```python
from build123d import *

# Parameters (mm, degrees)
SKETCH_1_W            = 100
SKETCH_1_H            = 62
SKETCH_1_W_2          = 110
SKETCH_1_H_2          = 30
EXTRUDE_467_DEPTH     = 2
SKETCH_2_R            = 1.25
CUT_EXTRUDE_872_DEPTH = 2
SKETCH_3_R            = 3.25
SKETCH_3_R_2          = 1.25
EXTRUDE_1188_DEPTH    = 3


with BuildPart() as part:
    # 草图1 → Extrude 467 (new body)
    with BuildSketch(Plane(origin=(0, 0, 0), x_dir=(1, 0, 0), z_dir=(0, 1, 0))):
        Rectangle(SKETCH_1_W, SKETCH_1_H)
        Rectangle(SKETCH_1_W_2, SKETCH_1_H_2)
    extrude(amount=EXTRUDE_467_DEPTH)

    # 草图2 → Cut-Extrude 872 (cut)
    with BuildSketch(Plane(origin=(0, 2, 0), x_dir=(1, 0, 0), z_dir=(0, 1, 0))):
        with Locations((-14, 24.5)):
            Circle(SKETCH_2_R)
        with Locations((44, 24.5)):
            Circle(SKETCH_2_R)
        with Locations((-14, -24.5)):
            Circle(SKETCH_2_R)
        with Locations((44, -24.5)):
            Circle(SKETCH_2_R)
    extrude(amount=-CUT_EXTRUDE_872_DEPTH, mode=Mode.SUBTRACT)

    # 草图3 → Extrude 1188 (add)
    with BuildSketch(Plane(origin=(0, 2, 0), x_dir=(1, 0, 0), z_dir=(0, 1, 0))):
        with Locations((-14, 24.5)):
            Circle(SKETCH_3_R)
        with Locations((-14, 24.5)):
            Circle(SKETCH_3_R_2, mode=Mode.SUBTRACT)
        with Locations((44, 24.5)):
            Circle(SKETCH_3_R)
        with Locations((44, 24.5)):
            Circle(SKETCH_3_R_2, mode=Mode.SUBTRACT)
        with Locations((-14, -24.5)):
            Circle(SKETCH_3_R)
        with Locations((-14, -24.5)):
            Circle(SKETCH_3_R_2, mode=Mode.SUBTRACT)
        with Locations((44, -24.5)):
            Circle(SKETCH_3_R)
        with Locations((44, -24.5)):
            Circle(SKETCH_3_R_2, mode=Mode.SUBTRACT)
    extrude(amount=EXTRUDE_1188_DEPTH)


solid = part.part
```
The listing builds one solid part. Answer for the finished solid, in the listing's coordinates (mm). A direction names the side the tool comes from. Give positions to 0.01 mm unless a question says otherwise; leave off trailing zeros. Order: outer loops, then holes, each group sorted by start corner. A loop starts at its lowest first (then second) coordinate and runs counter-clockwise, first axis right, second up. Notation, with made-up numbers: (41.25, -24) -> (99.25, -24) arc R12 cw to (99.25, -13) -> close; hole circle Ø3 at (7.5, -35). An arc over 180 degrees is marked (long way). One line per item, written item: value.
1) Find section C-C, the plane x = 44. Determine the outline of the cut face in (y, z).
Reported:
outline: (0, -31) -> (2, -31) -> (2, -27.75) -> (5, -27.75) -> (5, -25.75) -> (0, -25.75) -> close; (0, -23.25) -> (5, -23.25) -> (5, -21.25) -> (2, -21.25) -> (2, 21.25) -> (5, 21.25) -> (5, 23.25) -> (0, 23.25) -> close; (0, 25.75) -> (5, 25.75) -> (5, 27.75) -> (2, 27.75) -> (2, 31) -> (0, 31) -> close
2) Determine the mould class of faces 1 (the cylindrical face through (-16.579, 3.479, -22.522)), 2 (the flat face through (-50, 1, 23)), 3 (the flat face through (-1, 1, -31)), 4 (the flat face through (-53, 1, 15)) for opening direction Z: pulls with the +Z half, pulls with the -Z half, needs draft (parallel to the pull), parting line crosses it, or undercut.
Reported:
face 1: undercut
face 2: needs draft
face 3: pulls with the -Z half
face 4: pulls with the +Z half
3) Flat-ended cylindrical pins translate along their axes: P1, Ø2, axis at x = -14, z = 24.5, coming from the -Y side; P2, Ø0.6, axis at x = 52.5, y = 1, coming from the -Z side; P3, Ø1.6, axis at y = 0.5, z = 27, coming from the -X side; P4, Ø1, axis at x = -52, y = 1, coming from the +Z side. Find the tip coordinate at first contact, or state that the pin passes through.
Reported:
P1: passes through
P2: stops at z = -15
P3: stops at x = -50
P4: stops at z = 15
4) A tool of negligible diameter and unlimited length cuts with its end or side. For faces 5 (the cylindrical face through (47.002, 3.479, 25.745)), 6 (the flat face through (-1, 1, 31)), 7 (the flat face through (-14, 5, 26)), 8 (the flat face through (50, 1, -23)), 9 (the flat face through (-50, 1, -23)), from which of +Z, -Z, +X, -X, +Y, -Y can it reach the whole face along a straight path? Write none if from no direction.
Reported:
face 5: +Y
face 6: +Z, +X, -X, +Y, -Y
face 7: +Z, -Z, +X, -X, +Y
face 8: -Z, +X, +Y, -Y
face 9: -Z, -X, +Y, -Y
5) Find the intervals of material crossed by line 1 (Z direction, x = 44, y = 3.1); line 2 (X direction, y = 2.05, z = 24.5); line 3 (X direction, y = 1.05, z = 24.5), in increasing order.
Reported:
line 1: z = -27.75 to -25.75, -23.25 to -21.25, 21.25 to 23.25, 25.75 to 27.75
line 2: x = -17.25 to -15.25, -12.75 to -10.75, 40.75 to 42.75, 45.25 to 47.25
line 3: x = -50 to -15.25, -12.75 to 42.75, 45.25 to 50
6) Find section B-B, the plane z = 24.5. Determine the outline of the cut face in (x, y).
Reported:
outline: (-50, 0) -> (-15.25, 0) -> (-15.25, 5) -> (-17.25, 5) -> (-17.25, 2) -> (-50, 2) -> close; (-12.75, 0) -> (42.75, 0) -> (42.75, 5) -> (40.75, 5) -> (40.75, 2) -> (-10.75, 2) -> (-10.75, 5) -> (-12.75, 5) -> close; (45.25, 0) -> (50, 0) -> (50, 2) -> (47.25, 2) -> (47.25, 5) -> (45.25, 5) -> close
7) Find section A-A, the plane y = 1.25. Determine the outline of the cut face in (x, z), plus the area to 3 significant figures.
Reported:
outline: (-55, -15) -> (-50, -15) -> (-50, -31) -> (50, -31) -> (50, -15) -> (55, -15) -> (55, 15) -> (50, 15) -> (50, 31) -> (-50, 31) -> (-50, 15) -> (-55, 15) -> close; hole circle Ø2.5 at (-14, -24.5); hole circle Ø2.5 at (-14, 24.5); hole circle Ø2.5 at (44, -24.5); hole circle Ø2.5 at (44, 24.5)
area: 6,480 mm^2
8) Find section D-D, the plane z = 17. Determine the outline of the cut face in (x, y), plus the area to 3 significant figures.
Reported:
outline: (-50, 0) -> (50, 0) -> (50, 2) -> (-50, 2) -> close
area: 200 mm^2
